from build123d import *

# Parameters (mm, degrees)
SKETCH010_W     = 0.5
SKETCH010_H     = 5
POCKET001_DEPTH = 4
CHAMFER_SIZE    = 0.3


with BuildPart() as part:
    # Sketch008 → Revolution002 (revolve)
    with BuildSketch(Plane.XZ):
        Polygon((-3.6, 0), (-3.6, 2.452), (-4.699, 2.452), (-4.699, 5.5), (0, 5.5), (0, 4), (-1.3, 4), (-1.3, 1), (-2.3, 1), (-2.3, 4), (-3.1, 4), (-3.1, 0), align=None)
    revolve(axis=Axis((0, 0, 0), (0, 0, 1)))

    # Sketch010 → Pocket001 (cut)
    with BuildSketch(Plane.XY):
        Rectangle(SKETCH010_W, SKETCH010_H)
    extrude(amount=POCKET001_DEPTH, mode=Mode.SUBTRACT)

    # Chamfer
    chamfer_edges = [part.edges().sort_by_distance(p)[0] for p in [
        (4.699, 0, 5.5),
        (4.699, 0, 2.452),
        (1.3, 0, 1),
        (-1.003743, 0.826136, 1),
    ]]
    chamfer(chamfer_edges, length=CHAMFER_SIZE)


solid = part.part
Work out the finished part from the listing and answer in its coordinate system (mm). A direction names the side the tool comes from. Give positions to 0.01 mm unless a question says otherwise; leave off trailing zeros. Write each loop counter-clockwise with the first axis right and the second up, starting at its lowest first coordinate (ties: lowest second). Pieces come first, ordered by that corner, then holes.
Q1. The part is cut by section B-B on x = 0. Give the vertices of the cut face in (y, z), and give its area (3 significant figures).
Answer:
outline: (-4.7, 2.75) - (-4.4, 2.45) - (-3.6, 2.45) - (-3.6, 0) - (-3.1, 0) - (-3.1, 4) - (3.1, 4) - (3.1, 0) - (3.6, 0) - (3.6, 2.45) - (4.4, 2.45) - (4.7, 2.75) - (4.7, 5.2) - (4.4, 5.5) - (-4.4, 5.5) - (-4.7, 5.2) - close
area: 21.3 mm2
Q2. A tool of negligible diameter and unlimited length cuts with its end or side. For faces 4 (the face through (0.61, -4.66, 3.99)), 5 (the face through (1.3, 0, 2.6)), from which of +Z, -Z, +X, -X, +Y, -Y can it reach the whole face along a straight path? Write none if from no direction.
Answer:
face 4: +Z, -Z
face 5: -Z
Q3. Given pin 1 (0.8 mm diameter, centred on y = 2, z = 2, fed in from +X); pin 2 (1.1 mm diameter, centred on y = -1.5, z = 2.5, fed in from -X); pin 3 (2.5 mm diameter, centred on x = 1, y = 0.5, fed in from -Z), each flat-ended and moving along its own axis, determine where each tip first touches the part or whether it passes through.
Answer:
pin 1: stops at x = 3.22
pin 2: stops at x = -4.59
pin 3: stops at z = 1
Q4. The part is cut by section C-C on y = 0. Give the vertices of the cut face in (x, z).
Answer:
outline: (-4.7, 2.75) - (-4.4, 2.45) - (-3.6, 2.45) - (-3.6, 0) - (-3.1, 0) - (-3.1, 4) - (-2.3, 4) - (-2.3, 1) - (-1.6, 1) - (-1.3, 1.3) - (-1.3, 4) - (1.3, 4) - (1.3, 1.3) - (1.6, 1) - (2.3, 1) - (2.3, 4) - (3.1, 4) - (3.1, 0) - (3.6, 0) - (3.6, 2.45) - (4.4, 2.45) - (4.7, 2.75) - (4.7, 5.2) - (4.4, 5.5) - (-4.4, 5.5) - (-4.7, 5.2) - close
Q5. The part is cut by section A-A on z = 2.95. Give the vertices of the cut face in (x, y).
Answer:
outline: circle Ø9.4 at (0, 0); (-0.25, -2.29) - (-0.25, -1.28) arc R1.3 cw to (-0.25, 1.28) - (-0.25, 2.29) arc R2.3 ccw to start; (0.25, -2.29) arc R2.3 ccw to (0.25, 2.29) - (0.25, 1.28) arc R1.3 cw to (0.25, -1.28) - close; hole circle Ø6.2 at (0, 0)
Q6. Straight lines are drawn through the part: L1, parallel to X at y = 0, z = 1.7; L2, parallel to X at y = 0, z = 3.2; L3, parallel to Y at x = 0, z = 1.5. For each, find the intervals that lie inside material, in ascending order.
Answer:
L1: x = -3.6 to -3.1, -2.3 to -1.3, 1.3 to 2.3, 3.1 to 3.6
L2: x = -4.7 to -3.1, -2.3 to -1.3, 1.3 to 2.3, 3.1 to 4.7
L3: y = -3.6 to -3.1, 3.1 to 3.6
Q7. For a pull along X with two mould halves and no side action, classify faces 1 (the face through (0, 0, 5.5)), 2 (the face through (-3.434, -1.081, 1.243)), 3 (the face through (-1.3, 0, 2.6)) as released by +X, released by -X, zero draft, split by the parting line, or undercut.
Answer:
face 1: zero draft
face 2: split by the parting line
face 3: undercut
